from build123d import *

# Parameters (mm, degrees)
SKETCH1_W           = 26.3
SKETCH1_H           = 133
BOSS_EXTRUDE1_DEPTH = 5
SKETCH2_R           = 2.5
BOSS_EXTRUDE2_DEPTH = 5
BOSS_EXTRUDE3_START = -15
BOSS_EXTRUDE3_DEPTH = 103


with BuildPart() as part:
    # Sketch1 → Boss-Extrude1 (new body)
    with BuildSketch(Plane.XY):
        with Locations((-34.698380987, 507.595307356)):
            Rectangle(SKETCH1_W, SKETCH1_H)
        with BuildLine():
            ThreePointArc((-40.742130987, 444.245307356), (-43.767130987, 447.270307356), (-40.742130987, 450.295307356))
            Line((-40.742130987, 450.295307356), (-37.492130987, 450.295307356))
            ThreePointArc((-37.492130987, 450.295307356), (-34.467130987, 447.270307356), (-37.492130987, 444.245307356))
            Line((-37.492130987, 444.245307356), (-40.742130987, 444.245307356))
        make_face(mode=Mode.SUBTRACT)
        with BuildLine():
            ThreePointArc((-40.742130987, 460.120307356), (-43.767130987, 463.145307356), (-40.742130987, 466.170307356))
            Line((-40.742130987, 466.170307356), (-37.492130987, 466.170307356))
            ThreePointArc((-37.492130987, 466.170307356), (-34.467130987, 463.145307356), (-37.492130987, 460.120307356))
            Line((-37.492130987, 460.120307356), (-40.742130987, 460.120307356))
        make_face(mode=Mode.SUBTRACT)
        with BuildLine():
            ThreePointArc((-40.742130987, 475.995307356), (-43.767130987, 479.020307356), (-40.742130987, 482.045307356))
            Line((-40.742130987, 482.045307356), (-37.492130987, 482.045307356))
            ThreePointArc((-37.492130987, 482.045307356), (-34.467130987, 479.020307356), (-37.492130987, 475.995307356))
            Line((-37.492130987, 475.995307356), (-40.742130987, 475.995307356))
        make_face(mode=Mode.SUBTRACT)
        with BuildLine():
            ThreePointArc((-40.742130987, 488.695307356), (-43.767130987, 491.720307356), (-40.742130987, 494.745307356))
            Line((-40.742130987, 494.745307356), (-37.492130987, 494.745307356))
            ThreePointArc((-37.492130987, 494.745307356), (-34.467130987, 491.720307356), (-37.492130987, 488.695307356))
            Line((-37.492130987, 488.695307356), (-40.742130987, 488.695307356))
        make_face(mode=Mode.SUBTRACT)
        with BuildLine():
            ThreePointArc((-40.742130987, 504.570307356), (-43.767130987, 507.595307356), (-40.742130987, 510.620307356))
            Line((-40.742130987, 510.620307356), (-37.492130987, 510.620307356))
            ThreePointArc((-37.492130987, 510.620307356), (-34.467130987, 507.595307356), (-37.492130987, 504.570307356))
            Line((-37.492130987, 504.570307356), (-40.742130987, 504.570307356))
        make_face(mode=Mode.SUBTRACT)
        with BuildLine():
            ThreePointArc((-40.742130987, 520.445307356), (-43.767130987, 523.470307356), (-40.742130987, 526.495307356))
            Line((-40.742130987, 526.495307356), (-37.492130987, 526.495307356))
            ThreePointArc((-37.492130987, 526.495307356), (-34.467130987, 523.470307356), (-37.492130987, 520.445307356))
            Line((-37.492130987, 520.445307356), (-40.742130987, 520.445307356))
        make_face(mode=Mode.SUBTRACT)
        with BuildLine():
            ThreePointArc((-40.742130987, 533.057807356), (-43.767130987, 536.082807356), (-40.742130987, 539.107807356))
            Line((-40.742130987, 539.107807356), (-37.492130987, 539.107807356))
            ThreePointArc((-37.492130987, 539.107807356), (-34.467130987, 536.082807356), (-37.492130987, 533.057807356))
            Line((-37.492130987, 533.057807356), (-40.742130987, 533.057807356))
        make_face(mode=Mode.SUBTRACT)
        with BuildLine():
            ThreePointArc((-40.742130987, 548.932807356), (-43.767130987, 551.957807356), (-40.742130987, 554.982807356))
            Line((-40.742130987, 554.982807356), (-37.492130987, 554.982807356))
            ThreePointArc((-37.492130987, 554.982807356), (-34.467130987, 551.957807356), (-37.492130987, 548.932807356))
            Line((-37.492130987, 548.932807356), (-40.742130987, 548.932807356))
        make_face(mode=Mode.SUBTRACT)
        with BuildLine():
            ThreePointArc((-40.742130987, 564.707807356), (-43.867130987, 567.832807356), (-40.742130987, 570.957807356))
            Line((-40.742130987, 570.957807356), (-37.492130987, 570.957807356))
            ThreePointArc((-37.492130987, 570.957807356), (-34.367130987, 567.832807356), (-37.492130987, 564.707807356))
            Line((-37.492130987, 564.707807356), (-40.742130987, 564.707807356))
        make_face(mode=Mode.SUBTRACT)
    extrude(amount=BOSS_EXTRUDE1_DEPTH)



with BuildPart() as body_2:
    # Sketch2 → Boss-Extrude2 (new body)
    with BuildSketch(Plane.ZY.offset(21.548380987)):
        Polygon((0, 558.595307356), (0, 456.595307356), (0, 441.095307356), (-11.4, 441.095307356), (-11.4, 446.245307356), (-98.6, 446.245307356), (-98.6, 441.095307356), (-110, 441.095307356), (-110, 574.095307356), (-98.6, 574.095307356), (-98.6, 568.945307356), (-11.4, 568.945307356), (-11.4, 574.095307356), (0, 574.095307356), align=None)
        with Locations(Location((-5.7, 568.395307356, 0), (0, 0, 270))):
            Circle(SKETCH2_R, mode=Mode.SUBTRACT)
        with Locations(Location((-104.3, 568.395307356, 0), (0, 0, 270))):
            Circle(SKETCH2_R, mode=Mode.SUBTRACT)
        with Locations(Location((-104.3, 446.795307356, 0), (0, 0, 270))):
            Circle(SKETCH2_R, mode=Mode.SUBTRACT)
        with Locations(Location((-5.7, 446.795307356, 0), (0, 0, 270))):
            Circle(SKETCH2_R, mode=Mode.SUBTRACT)
    extrude(amount=BOSS_EXTRUDE2_DEPTH)


with BuildPart() as part_1:
    add(part.part)

    add(body_2.part)  # Boss-Extrude3 merges body 2
    # Sketch4 → Boss-Extrude3 (add)
    with BuildSketch(Plane(origin=(0, 574.095307356, 0), x_dir=(1, 0, 0), z_dir=(0, 1, 0)).offset(BOSS_EXTRUDE3_START)):
        Polygon((-26.548380987, 0), (-29.548380987, 0), (-26.548380987, 10), align=None)
    extrude(amount=-BOSS_EXTRUDE3_DEPTH)


solid = part_1.part
CAD build for the part. Positions are in the model's coordinates, mm. A direction names the side the tool comes from. Round coordinates to 2 decimals unless told otherwise and drop trailing zeros. Order: outer loops, then holes, each group sorted by start corner. A loop starts at its lowest first (then second) coordinate and runs counter-clockwise, first axis right, second up. Notation, with made-up numbers: M 68.5,18 L 106.5,18 A37 cw 106.5,56 Z; hole C 26,10 d6. An arc over 180 degrees is marked long. Use one line per item in the form item = value.
Q1. Flat gauge pins, fed straight in: P1, Ø12, axis at y = 556, z = -28, coming from the -X side; P2, Ø2, axis at x = -45, y = 523.5, coming from the -Z side; P3, Ø4, axis at x = -23.5, z = -57, coming from the +Y side. Where does each tip first touch, or does it go through?
Recorded:
P1 = -26.55
P2 = 0
P3 = 568.95
Q2. Saw through at D-D on x = -31.75. Give the cut face in (y, z), then the cut area to 3 significant figures.
Recorded:
outline = M 441.1,0 L 574.1,0 L 574.1,5 L 441.1,5 Z
area = 665 mm^2
Q3. Saw through at B-B on y = 478. Give the cut face in (x, z), then the cut area to 3 significant figures.
Recorded:
outline = M -47.85,0 L -43.59,0 L -43.59,5 L -47.85,5 Z; M -34.64,0 L -29.55,0 L -26.55,-10 L -26.55,-110 L -21.55,-110 L -21.55,5 L -34.64,5 Z
area = 652 mm^2
Q4. Saw through at C-C on y = 563. Give the cut face in (x, z), then the cut area to 4 significant figures.
Recorded:
outline = M -47.85,0 L -26.55,0 L -26.55,-110 L -21.55,-110 L -21.55,5 L -47.85,5 Z
area = 681.5 mm^2
Q5. Two-plate mould, pull along Z, no slides. Class faces 1 (the flat face through (-39, 482.045, 2)), 2 (the flat face through (-24, 507, -110)), 3 (the cylindrical face through (-24.013, 444.486, -6.658)), 4 (the flat face through (-24, 571, -11.4)): +Z half, -Z half, draft (parallel to the pull), parting line (faces both ways), or undercut.
Recorded:
face_1 = draft
face_2 = -Z half
face_3 = undercut
face_4 = undercut
Q6. Which spindle directions (+Z, -Z, +X, -X, +Y, -Y) get a long thin tool onto all of the face, cutting with end or side? Do faces 5 (the cylindrical face through (-43.766, 523.404, 2.465)), 6 (the cylindrical face through (-24.013, 570.893, -104.19)). Say none if no direction does.
Recorded:
face_5 = +Z, -Z
face_6 = +X, -X
Q7. Saw through at A-A on z = -104.3. Give the cut face in (x, y), then the cut area to 3 significant figures.
Recorded:
outline = M -26.55,441.1 L -21.55,441.1 L -21.55,444.3 L -26.55,444.3 Z; M -26.55,449.3 L -21.55,449.3 L -21.55,565.9 L -26.55,565.9 Z; M -26.55,570.9 L -21.55,570.9 L -21.55,574.1 L -26.55,574.1 Z
area = 615 mm^2
Q8. Probe L1, parallel to Z at x = -44.25, y = 544.5; L2, parallel to X at y = 479.5, z = -61.5; L3, parallel to Y at x = -26, z = -89. List the from-to ranges inside material, lowest first.
Recorded:
L1 = 0 to 5
L2 = -26.55 to -21.55
L3 = 446.25 to 568.95
